```python
from build123d import *

# Parameters (mm, degrees)
SKETCH_1_W      = 56
SKETCH_1_H      = 30
EXTRUDE_1_DEPTH = 8
FILLET_1_R      = 1


with BuildPart() as part:
    # 草图1 → 凸台-拉伸1 (new body)
    with BuildSketch(Plane.XY):
        with Locations((13, -0.54396632)):
            Rectangle(SKETCH_1_W, SKETCH_1_H)
        with BuildLine():
            Line((0, 9), (28, 9))
            ThreePointArc((28, 9), (37, 0), (28, -9))
            Line((28, -9), (22, -9))
            Line((22, -9), (19.655104495, -11.8))
            Line((19.655104495, -11.8), (8.344895505, -11.8))
            Line((8.344895505, -11.8), (6, -9))
            Line((6, -9), (0, -9))
            ThreePointArc((0, -9), (-9, 0), (0, 9))
        make_face(mode=Mode.SUBTRACT)
    extrude(amount=EXTRUDE_1_DEPTH)

    # 圆角1
    fillet_1_edges = [part.edges().sort_by_distance(p)[0] for p in [
        (6, -9, 4),
        (8.344895505, -11.8, 4),
        (19.655104495, -11.8, 4),
        (22, -9, 4),
    ]]
    fillet(fillet_1_edges, radius=FILLET_1_R)


solid = part.part
```
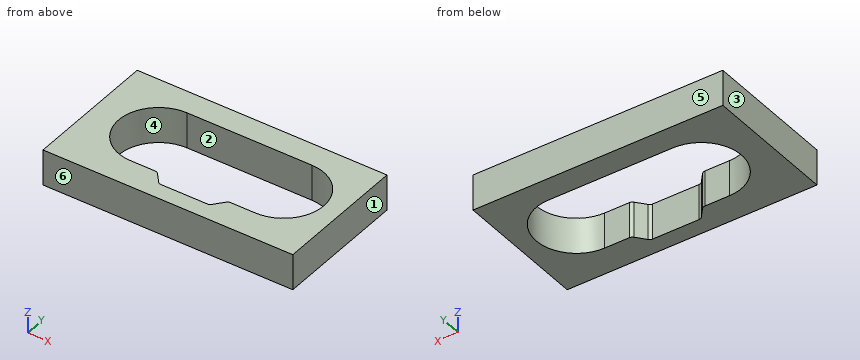
Verification items for the finished model (mm, model axes). Face numbers are marked on the shaded views. A direction names the side the tool comes from. Round coordinates to 2 decimals unless told otherwise and drop trailing zeros. Write each loop counter-clockwise with the first axis right and the second up, starting at its lowest first coordinate (ties: lowest second). Pieces come first, ordered by that corner, then holes.
1. Gauge pin test, flat end, axial feed: P1, Ø3, axis at x = 33.5, y = 2.5, coming from the -Z side. Record the tip position at first contact, or that the pin passes through.
2. Section check B-B on x = 13. Enter the section's corners in (y, z).
3. Scan lines: L1, parallel to Y at x = 16, z = 2.75; L2, parallel to Y at x = 25.5, z = 1.5; L3, parallel to X at y = -8, z = 3.5. Record each from-to range of solid material in increasing order.
4. Access from +Z, -Z, +X, -X, +Y, -Y to the whole of each face (thin tool, end or side, straight path). Record for the marked faces 1 and 2.
5. Section check C-C on z = 7. Enter the section's corners in (x, y), plus the area to 3 significant figures.
6. Draft check along Y on the marked faces 3, 4, 5 and 6. Enter one of: +Y half, -Y half, draft (parallel to the pull), parting line (faces both ways), or undercut.
7. Section check A-A on y = 0. Enter the section's corners in (x, z).
Answer:
1. P1: passes through
2. outline: (-15.54, 0) - (-11.8, 0) - (-11.8, 8) - (-15.54, 8) - close; (9, 0) - (14.46, 0) - (14.46, 8) - (9, 8) - close
3. L1: y = -15.54 to -11.8, 9 to 14.46
3. L2: y = -15.54 to -9, 9 to 14.46
3. L3: x = -15 to -4.12, 32.12 to 41
4. face 1: +Z, -Z, +X, +Y, -Y
4. face 2: +Z, -Z
5. outline: (-15, -15.54) - (41, -15.54) - (41, 14.46) - (-15, 14.46) - close; hole (0, -9) - (5.53, -9) arc R1 cw to (6.3, -9.36) - (8.05, -11.44) arc R1 ccw to (8.81, -11.8) - (19.19, -11.8) arc R1 ccw to (19.95, -11.44) - (21.7, -9.36) arc R1 cw to (22.47, -9) - (28, -9) arc R9 ccw to (28, 9) - (0, 9) arc R9 ccw to start
5. area: 883 mm2
6. face 3: draft
6. face 4: undercut
6. face 5: +Y half
6. face 6: -Y half
7. outline: (-15, 0) - (-9, 0) - (-9, 8) - (-15, 8) - close; (37, 0) - (41, 0) - (41, 8) - (37, 8) - close
